Design review of the part built by this model. Coordinates are the model's own, in mm. A direction names the side the tool comes from. Give positions to 0.01 mm unless a question says otherwise; leave off trailing zeros. Write each loop counter-clockwise with the first axis right and the second up, starting at its lowest first coordinate (ties: lowest second). Pieces come first, ordered by that corner, then holes. Notation, with made-up numbers: M -25,-7 L 29,-7 A9 cw 29,3 Z; hole C 65.25,27 d9. An arc over 180 degrees is marked long. Write each question's results on one line, items separated by ' | '. Start each with the question number.
from build123d import *

# Parameters (mm, degrees)
PAD001_DEPTH         = 20.5
POCKET_DEPTH         = 17.8
SKETCH020_W          = 89.65
SKETCH020_H          = 5
POCKET002_DEPTH      = 12.8
HOLE006_D            = 5.3
HOLE006_CBORE_D      = 8.9
HOLE006_CBORE_DEPTH  = 5.4
SKETCH032_W          = 35
SKETCH032_H          = 37
POCKET010_DEPTH      = 102.001
SKETCH033_W          = 5
SKETCH033_H          = 15
POCKET011_DEPTH      = 20.501
POCKET011_DEPTH_BACK = 20.501
SKETCH034_R          = 1.5
POCKET012_DEPTH      = 103.501


with BuildPart() as part:
    # Sketch018 → Pad001 (new body, symmetric)
    with BuildSketch(Plane.XZ):
        Polygon((71.9, 102.9), (-23.5, 7.5), (-23.5, 0), (71.9, 0), (71.9, -10), (79.9, -10), (79.9, 102.9), align=None)
    extrude(amount=PAD001_DEPTH, both=True)

    # Sketch019 → Pocket (cut, symmetric)
    with BuildSketch(Plane.XZ):
        Polygon((-17.5, 4.5), (71.9, 4.5), (71.9, 104.5), (-27.5, 104.5), (-27.5, 14.5), align=None)
    extrude(amount=POCKET_DEPTH, both=True, mode=Mode.SUBTRACT)

    # Sketch020 → Pocket002 (cut, symmetric)
    with BuildSketch(Plane.XZ):
        with Locations((27.075, 2.5)):
            Rectangle(SKETCH020_W, SKETCH020_H)
    extrude(amount=POCKET002_DEPTH, both=True, mode=Mode.SUBTRACT)

    # Hole006 (through all)
    with Locations(Plane(origin=(71.9, 0, 0), x_dir=(0, 1, 0), z_dir=(-1, 0, 0))):
        with Locations((-12.5, -97), (12.5, -97), (-12.5, 5), (12.5, 5)):
            CounterBoreHole(HOLE006_D / 2, HOLE006_CBORE_D / 2, HOLE006_CBORE_DEPTH)

    # Sketch032 → Pocket010 (cut, through all)
    with BuildSketch(Plane.YZ.offset(78.5)):
        with Locations((0, 39.3)):
            Rectangle(SKETCH032_W, SKETCH032_H)
    extrude(amount=-POCKET010_DEPTH, mode=Mode.SUBTRACT)

    # Sketch033 → Pocket011 (cut, two sides)
    with BuildSketch(Plane.XZ) as pocket011_sk:
        with Locations((74.4, 41.5)):
            Rectangle(SKETCH033_W, SKETCH033_H)
    extrude(amount=-POCKET011_DEPTH, mode=Mode.SUBTRACT)
    extrude(pocket011_sk.sketch, amount=POCKET011_DEPTH_BACK, mode=Mode.SUBTRACT)

    # Sketch034 → Pocket012 (cut, through all)
    with BuildSketch(Plane.YZ.offset(80)):
        with Locations((-12.75, 52.94381)):
            Circle(SKETCH034_R)
        with Locations((12.75, 52.94381)):
            Circle(SKETCH034_R)
        with Locations((12.75, 25.94381)):
            Circle(SKETCH034_R)
        with Locations((-12.75, 25.94381)):
            Circle(SKETCH034_R)
        with BuildLine():
            ThreePointArc((-13.401099, 46.669643), (-14.401099, 47.669643), (-15.401099, 46.669643))
            Line((-15.401099, 46.669643), (-15.401099, 36.32))
            ThreePointArc((-15.401099, 36.32), (-14.401099, 35.32), (-13.401099, 36.32))
            Line((-13.401099, 46.669643), (-13.401099, 36.32))
        make_face()
        with BuildLine():
            ThreePointArc((15.401099, 46.669643), (14.401099, 47.669643), (13.401099, 46.669643))
            Line((13.401099, 46.669643), (13.401099, 36.32))
            ThreePointArc((13.401099, 36.32), (14.401099, 35.32), (15.401099, 36.32))
            Line((15.401099, 46.669643), (15.401099, 36.32))
        make_face()
    extrude(amount=-POCKET012_DEPTH, mode=Mode.SUBTRACT)


solid = part.part
Q1. Wall thickness on line 1 along Y through (x, z) = (78.85, 97); line 2 along Z through (x, y) = (77.9, -12.5); line 3 along Y through (x, z) = (74, 97): over which ranges is each line inside the solid? List them lowest first. Write a range as from..to.
Q2. We need section A-A on z = 97. Write out the cut boundary in (x, y), and give its area (3 significant figures).
Q3. The part is to be moulded in two halves that separate along Z. For faces 1 (the cylindrical face through (79.21, -13.856, 53.958)), 2 (the flat face through (74, 19, 49)), 3 (the flat face through (35, 17.8, 33)), 4 (the flat face through (27, -15, 4.5)), say which applies: pulls with the +Z half, pulls with the -Z half, needs draft (parallel to the pull), parting line crosses it, or undercut.
Q4. We need section B-B on x = 12. Write out the cut boundary in (y, z), and give its area (3 significant figures).
Q5. For pin 1 Ø1.8 at (y, z) = (12.75, 52.94) entering from -X; pin 2 Ø7 at (y, z) = (-12.5, 97) entering from -X; pin 3 Ø1.5 at (x, y) = (-10, -13.5) entering from +Z; pin 4 Ø4 at (x, y) = (-10.5, 11) entering from -Z, all flat-tipped, find the tip position at first contact; note any pin that passes through.
Q6. We need section C-C on y = -2. Write out the cut boundary in (x, z).
Q7. For faces 5 (the cylindrical face through (74.562, -8.389, -3.296)), 6 (the flat face through (-20, 0, 7)), 7 (the flat face through (-17.75, 0, 2)), list the 3-axis set-ups (+Z, -Z, +X, -X, +Y, -Y) from which the entire face can be reached by the end or side of a thin tool; tool diameter is ignored.
Q8. We need section D-D on z = 77.5. Write out the cut boundary in (x, y).
Answer sheet:
1) line 1: -20.5..-15.15, -9.85..9.85, 15.15..20.5 | line 2: -10..-7.65, -2.35..20.8, 57.8..94.35, 99.65..102.9 | line 3: -20.5..-16.95, -8.05..8.05, 16.95..20.5
2) outline: M 66,-20.5 L 79.9,-20.5 L 79.9,-15.15 L 77.3,-15.15 L 77.3,-16.95 L 71.9,-16.95 L 71.9,-17.8 L 66,-17.8 Z; M 66,17.8 L 71.9,17.8 L 71.9,16.95 L 77.3,16.95 L 77.3,15.15 L 79.9,15.15 L 79.9,20.5 L 66,20.5 Z; M 71.9,-8.05 L 77.3,-8.05 L 77.3,-9.85 L 79.9,-9.85 L 79.9,9.85 L 77.3,9.85 L 77.3,8.05 L 71.9,8.05 Z | area: 236 mm^2
3) face 1: undercut | face 2: undercut | face 3: needs draft | face 4: pulls with the +Z half
4) outline: M -20.5,0 L -12.8,0 L -12.8,4.5 L -17.8,4.5 L -17.8,43 L -20.5,43 Z; M 12.8,0 L 20.5,0 L 20.5,43 L 17.8,43 L 17.8,4.5 L 12.8,4.5 Z | area: 277 mm^2
5) pin 1: through | pin 2: x = 77.3 | pin 3: z = 4.5 | pin 4: z = 0
6) outline: M -23.5,0 L -17.75,0 L -17.75,4.75 L -22,9 L -23.5,7.5 Z; M 71.9,-10 L 79.9,-10 L 79.9,102.9 L 71.9,102.9 L 71.9,57.8 L 78.5,57.8 L 78.5,20.8 L 71.9,20.8 Z
7) face 5: -X | face 6: +Z | face 7: +Z, -Z
8) outline: M 46.5,-20.5 L 79.9,-20.5 L 79.9,20.5 L 46.5,20.5 L 46.5,17.8 L 71.9,17.8 L 71.9,-17.8 L 46.5,-17.8 Z
